```python
from build123d import *

# Parameters (mm, degrees)
F0_R     = 25.4
F1_DEPTH = 12.7
F3_DEPTH = 12.7
F4_R     = 3.302
F5_DEPTH = 12.7


with BuildPart() as f1:
    # F0 (on Front) → F1 (new body)
    with BuildSketch(Plane.XZ):
        Circle(F0_R)
    extrude(amount=F1_DEPTH)

    # F2 (on Front) → F3 (join)
    with BuildSketch(Plane.XZ):
        Polygon((-21.703257, 13.880826), (-27.935632, 12.664274), (-23.76588, 7.875155), align=None)
        Polygon((-30.501175, 3.234462), (-25.036675, 0), (-24.967798, 6.349626), align=None)
        Polygon((-16.235516, 20.002918), (-22.534213, 20.808476), (-20.082498, 14.950866), align=None)
        Polygon((-9.119631, 24.094419), (-14.845239, 26.840311), (-14.360447, 20.508844), align=None)
        Polygon((-1.07797, 25.739982), (-5.649254, 30.14746), (-7.180599, 23.984872), align=None)
        Polygon((7.073122, 24.772559), (4.120212, 30.394198), (0.728185, 25.026084), align=None)
        Polygon((14.506187, 21.290356), (13.471417, 27.555477), (8.563047, 23.526779), align=None)
        Polygon((20.466661, 15.646868), (21.455074, 21.919471), (15.528635, 19.63916), align=None)
        Polygon((24.349468, 8.414994), (27.260726, 14.058315), (20.917837, 13.757878), align=None)
        Polygon((25.760446, 0.328874), (30.299013, 4.770034), (24.183571, 6.479968), align=None)
    extrude(amount=F3_DEPTH)

    # F4 (on face) → F5 (cut)
    with BuildSketch(Plane.XZ.offset(12.7)):
        Circle(F4_R)
    extrude(amount=-F5_DEPTH, mode=Mode.SUBTRACT)


solid = f1.part
```
Design review of the part built by this model. Coordinates are the model's own, in mm. A direction names the side the tool comes from. Coordinates: 2 decimals unless noted, no trailing zeros. Loops run counter-clockwise (first coordinate to the right, second up) from the corner with the lowest first, then second, coordinate; pieces in that order, holes last. Notation, with made-up numbers: (36, 52) -> (58, 52) arc R28 cw to (58, 73) -> close; hole circle Ø3 at (73.5, 42). An arc over 180 degrees is marked (long way). Answer as a JSON object with one key per item and string values.
Q1. Take a section at A-A on x = 0. Give the boundary of the cut face in (y, z).
Answer block:
{"outline": "(-12.7, -25.4) -> (0, -25.4) -> (0, -3.3) -> (-12.7, -3.3) -> close; (-12.7, 3.3) -> (0, 3.3) -> (0, 25.4) -> (-12.7, 25.4) -> close"}
Q2. Take a section at B-B on z = -2. Give the boundary of the cut face in (x, y), plus the area to 3 significant figures.
Answer block:
{"outline": "(-25.32, -12.7) -> (-2.63, -12.7) -> (-2.63, 0) -> (-25.32, 0) -> close; (2.63, -12.7) -> (25.32, -12.7) -> (25.32, 0) -> (2.63, 0) -> close", "area": "576 mm^2"}
Q3. Take a section at C-C on z = -20. Give the boundary of the cut face in (x, y), plus the area to 3 significant figures.
Answer block:
{"outline": "(-15.66, -12.7) -> (15.66, -12.7) -> (15.66, 0) -> (-15.66, 0) -> close", "area": "398 mm^2"}
Q4. Clearance check with flat-ended pins moving along their axes: pin 1 Ø1.5 at (x, y) = (-21, -4) entering from -Z; pin 2 Ø2 at (y, z) = (-9.5, 16) entering from +X; pin 3 Ø5 at (x, y) = (-20, -10) entering from +Z. State where each tip first meets the part, or that it passes through.
Answer block:
{"pin 1": "stops at z = -15.33", "pin 2": "stops at x = 20.68", "pin 3": "stops at z = 20.8"}
Q5. Tool access review of faces 1 (the flat face through (6, -12.7, 3)), 2 (the flat face through (25.785, -6.261, 11.197)), 3 (the flat face through (-27.7, -6.26, 4.81)), 4 (the flat face through (-6.354, -6.261, 27.311)): name each direction out of +Z, -Z, +X, -X, +Y, -Y from which nothing blocks a thin tool from reaching the whole face with its end or side.
Answer block:
{"face 1": "+Z, -Z, +X, -X, -Y", "face 2": "+X, +Y, -Y", "face 3": "-X, +Y, -Y", "face 4": "+Z, +Y, -Y"}
Q6. The part is to be moulded in two halves that separate along Z. For faces 5 (the cylindrical face through (3.05, -6.44, -1.26)), 6 (the flat face through (6, 0, 3)), 7 (the flat face through (18.73, -6.26, 20.87)), say which applies: +Z half, -Z half, draft (parallel to the pull), parting line (faces both ways), or undercut.
Answer block:
{"face 5": "undercut", "face 6": "draft", "face 7": "+Z half"}
Q7. To check wall thickness, follow L1, parallel to Z at x = 0, y = -6; L2, parallel to X at y = -0.75, z = 27; L3, parallel to Z at x = 12.5, y = -9. State the ranges of each line that lie inside material, in increasing order.
Answer block:
{"L1": "z = -25.4 to -3.3, 3.3 to 25.4", "L2": "x = -6.43 to -2.38, 1.98 to 5.9, 12.79 to 13.56", "L3": "z = -22.11 to 26.76"}
